Work out the finished part from the listing and answer in its coordinate system (mm). Face numbers are marked on the shaded views. Coordinates: 2 decimals unless noted, no trailing zeros. Loops run counter-clockwise (first coordinate to the right, second up) from the corner with the lowest first, then second, coordinate; pieces in that order, holes last. Notation, with made-up numbers: (82, -7) -> (141, -7) arc R23 ccw to (141, 3) -> close; hole circle Ø4 at (-33.5, 54). An arc over 180 degrees is marked (long way). Answer as CSV lines item,"result".
```python
from build123d import *

# Parameters (mm, degrees)
F0_W     = 6.5
F0_H     = 30
F1_DEPTH = 495
F3_D     = 4.1


with BuildPart() as f1:
    # F0 (on Front) → F1 (new body)
    with BuildSketch(Plane.XZ):
        with Locations((14.25, 36)):
            Rectangle(F0_W, F0_H)
        with Locations((65.75, 36)):
            Rectangle(F0_W, F0_H)
        Polygon((0, 21), (0, 0), (80, 0), (80, 21), (69, 21), (62.5, 21), (62.5, 8), (17.5, 8), (17.5, 21), (11, 21), align=None)
    extrude(amount=F1_DEPTH)

    # F3 (through all)
    with Locations(Plane.XY.offset(21)):
        with Locations((75, -22.5), (75, -72.5), (75, -122.5), (75, -172.5), (75, -222.5), (75, -272.5), (75, -322.5), (75, -372.5), (75, -422.5), (75, -472.5), (5, -22.5), (5, -72.5), (5, -122.5), (5, -172.5), (5, -222.5), (5, -272.5), (5, -322.5), (5, -372.5), (5, -422.5), (5, -472.5)):
            Hole(F3_D / 2)


solid = f1.part
```
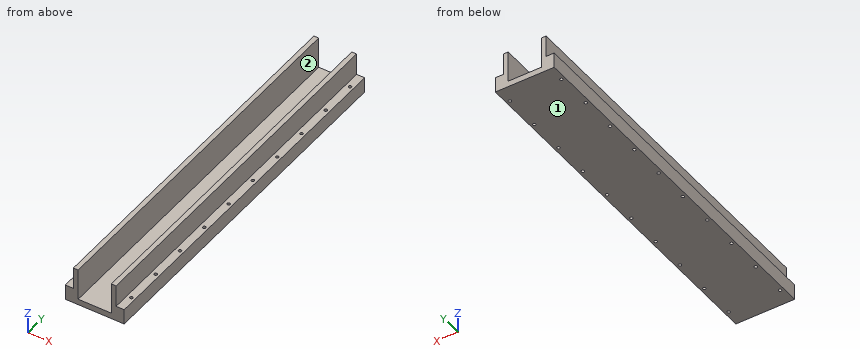
(1) Consider line 1 along X through (y, z) = (-422.5, 17); line 2 along X through (y, z) = (-123, 39); line 3 along X through (y, z) = (-345, 13.5). Determine where each line is inside the solid, lowest interval first.
Computed values:
line 1,"0 to 2.95, 7.05 to 17.5, 62.5 to 72.95, 77.05 to 80"
line 2,"11 to 17.5, 62.5 to 69"
line 3,"0 to 17.5, 62.5 to 80"
(2) For a pull along X with two mould halves and no side action, classify the marked faces 1 and 2 as pulls with the +X half, pulls with the -X half, needs draft (parallel to the pull), parting line crosses it, or undercut.
Computed values:
face 1,"needs draft"
face 2,"undercut"
(3) Flat-ended cylindrical pins translate along their axes: pin 1 Ø6.5 at (x, y) = (75, -172.5) entering from +Z; pin 2 Ø3.5 at (x, y) = (5, -272.5) entering from -Z; pin 3 Ø4 at (x, y) = (54, -77.5) entering from +Z; pin 4 Ø12 at (y, z) = (-198, 43.5) entering from -X. Find the tip coordinate at first contact, or state that the pin passes through.
Computed values:
pin 1,"z = 21"
pin 2,"through"
pin 3,"z = 8"
pin 4,"x = 11"
(4) A cutting plane is placed at D-D, the plane x = 42.5. Write down the section's boundary in (y, z), and give its area (3 significant figures).
Computed values:
outline,"(-495, 0) -> (0, 0) -> (0, 8) -> (-495, 8) -> close"
area,"3,960 mm2"
(5) A cutting plane is placed at C-C, the plane y = -257. Write down the section's boundary in (x, z), and give its area (4 significant figures).
Computed values:
outline,"(0, 0) -> (80, 0) -> (80, 21) -> (69, 21) -> (69, 51) -> (62.5, 51) -> (62.5, 8) -> (17.5, 8) -> (17.5, 51) -> (11, 51) -> (11, 21) -> (0, 21) -> close"
area,"1,485 mm2"
(6) A cutting plane is placed at A-A, the plane z = 14.5. Count the separate pieces of the cut face and the enclosed holes in it, and give its area (3 significant figures).
Computed values:
separate pieces,"2"
enclosed holes,"20"
area,"17,100 mm2"
(7) A cutting plane is placed at B-B, the plane z = 42.5. Write down the section's boundary in (x, y), and give its area (4 significant figures).
Computed values:
outline,"(11, -495) -> (17.5, -495) -> (17.5, 0) -> (11, 0) -> close; (62.5, -495) -> (69, -495) -> (69, 0) -> (62.5, 0) -> close"
area,"6,435 mm2"
